CAD build for the part. Positions are in the model's coordinates, mm. Face numbers are marked on the shaded views. A direction names the side the tool comes from. Round coordinates to 2 decimals unless told otherwise and drop trailing zeros. Loops run counter-clockwise (first coordinate to the right, second up) from the corner with the lowest first, then second, coordinate; pieces in that order, holes last.
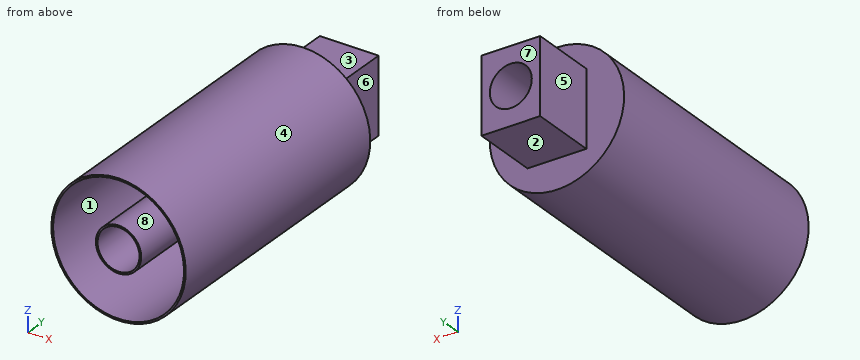
from build123d import *

# Parameters (mm, degrees)
SKETCH_1_R          = 40
EXTRUDE_1_DEPTH     = 160
SKETCH_2_W          = 35
SKETCH_2_H          = 45
EXTRUDE_2_DEPTH     = 40
SKETCH_7_R          = 12.5
CUT_EXTRUDE_2_DEPTH = 208.846096908
SHELL_1_T           = -1


with BuildPart() as part:
    # Эскиз1 → Бобышка-Вытянуть1 (new body)
    with BuildSketch(Plane(origin=(0, 0, 0), x_dir=(1, 0, 0), z_dir=(0, 1, 0))):
        with Locations(Location((0, 0, 0), (0, 0, 270))):
            Circle(SKETCH_1_R)
    extrude(amount=EXTRUDE_1_DEPTH)

    # Эскиз2 → Бобышка-Вытянуть2 (add)
    with BuildSketch(Plane(origin=(0, 160, 0), x_dir=(1, 0, 0), z_dir=(0, 1, 0))):
        Rectangle(SKETCH_2_W, SKETCH_2_H)
    extrude(amount=EXTRUDE_2_DEPTH)

    # Эскиз7 → Вырез-Вытянуть2 (cut, through all)
    with BuildSketch(Plane(origin=(0, 200, 0), x_dir=(1, 0, 0), z_dir=(0, 1, 0))):
        with Locations(Location((0, 0, 0), (0, 0, 270))):
            Circle(SKETCH_7_R)
    extrude(amount=-CUT_EXTRUDE_2_DEPTH, mode=Mode.SUBTRACT)

    # Оболочка1
    shell_1_openings = [part.faces().sort_by_distance(p)[0] for p in [
        (0, 0, -38.86862915),
    ]]
    offset(amount=SHELL_1_T, openings=shell_1_openings, kind=Kind.INTERSECTION)


solid = part.part
Item 1: Cut at D-D (y = 79). List the corners of the cut face in (x, z), plus the area to 3 significant figures.
Verdict:
outline: circle Ø80 at (0, 0); circle Ø27 at (0, 0); hole circle Ø78 at (0, 0); hole circle Ø25 at (0, 0)
area: 330 mm2
Item 2: Cut at C-C (x = -9). List the corners of the cut face in (y, z).
Verdict:
outline: (0, -38.97) - (160, -38.97) - (160, -22.5) - (200, -22.5) - (200, -8.67) - (0, -8.67) - (0, -10.06) - (199, -10.06) - (199, -21.5) - (159, -21.5) - (159, -37.95) - (0, -37.95) - close; (0, 8.67) - (200, 8.67) - (200, 22.5) - (160, 22.5) - (160, 38.97) - (0, 38.97) - (0, 37.95) - (159, 37.95) - (159, 21.5) - (199, 21.5) - (199, 10.06) - (0, 10.06) - close
Item 3: Flat gauge pins, fed straight in: P1, Ø1, axis at x = 31.5, z = 24, coming from the +Y side; P2, Ø6, axis at x = 11, y = 163.5, coming from the -Z side; P3, Ø3, axis at x = 27, y = 61, coming from the -Z side. Where does each tip first touch, or does it go through?
Verdict:
P1: stops at y = 160
P2: stops at z = -22.5
P3: stops at z = -30.82
Item 4: Wall check: L1, parallel to X at y = 92.5, z = 0; L2, parallel to Z at x = -3.5, y = 93.5; L3, parallel to X at y = 141, z = 3. Give the ranges that are in metal, low to high.
Verdict:
L1: x = -40 to -39, -13.5 to -12.5, 12.5 to 13.5, 39 to 40
L2: z = -39.85 to -38.84, -13.04 to -12, 12 to 13.04, 38.84 to 39.85
L3: x = -39.89 to -38.88, -13.16 to -12.13, 12.13 to 13.16, 38.88 to 39.89
Item 5: Cut at A-A (z = 0). List the corners of the cut face in (x, y).
Verdict:
outline: (-40, 0) - (-39, 0) - (-39, 159) - (-16.5, 159) - (-16.5, 199) - (-13.5, 199) - (-13.5, 0) - (-12.5, 0) - (-12.5, 200) - (-17.5, 200) - (-17.5, 160) - (-40, 160) - close; (12.5, 0) - (13.5, 0) - (13.5, 199) - (16.5, 199) - (16.5, 159) - (39, 159) - (39, 0) - (40, 0) - (40, 160) - (17.5, 160) - (17.5, 200) - (12.5, 200) - close
Item 6: Mould opens along Z. For the marked faces 1, 2 and 3 say: released by +Z, released by -Z, zero draft, split by the parting line, or undercut.
Verdict:
face 1: undercut
face 2: released by -Z
face 3: released by +Z
Item 7: Cut at B-B (y = 169). List the corners of the cut face in (x, z), plus the area to 3 significant figures.
Verdict:
outline: (-17.5, -22.5) - (17.5, -22.5) - (17.5, 22.5) - (-17.5, 22.5) - close; circle Ø27 at (0, 0); hole (-16.5, -21.5) - (16.5, -21.5) - (16.5, 21.5) - (-16.5, 21.5) - close; hole circle Ø25 at (0, 0)
area: 238 mm2
Item 8: 3-axis set-ups, long thin cutter, end or side, ignore diameter. For the marked faces 4, 5, 6, 7 and 8: which of +Z, -Z, +X, -X, +Y, -Y reach the whole face in a straight line?
Verdict:
face 4: +Y, -Y
face 5: +Z, -Z, -X, +Y
face 6: +Z, -Z, +X, +Y
face 7: +Z, -Z, +X, -X, +Y
face 8: -Y
